Input: part model. Units: mm. Frame: model coordinates. Face numbers are marked on the shaded views. Coordinates: 2 decimals unless noted, no trailing zeros. Write each loop counter-clockwise with the first axis right and the second up, starting at its lowest first coordinate (ties: lowest second). Pieces come first, ordered by that corner, then holes. Notation, with made-up numbers: M 65.25,-0.75 L 100.25,-0.75 A11 cw 100.25,20.25 Z; hole C 8,-23 d9. An arc over 180 degrees is marked long. Use one line per item in the form item = value.
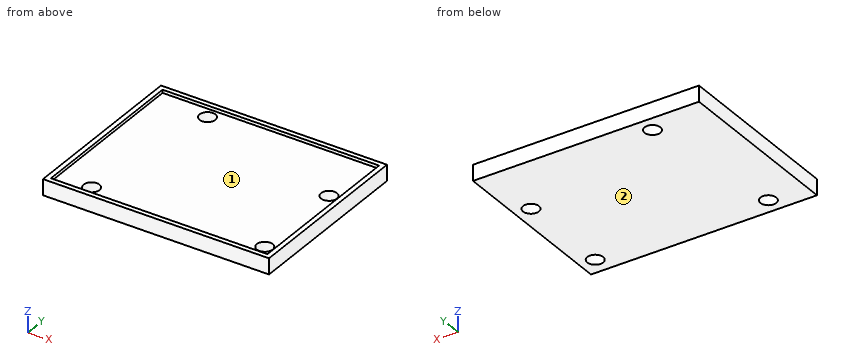
from build123d import *

# Parameters (mm, degrees)
SKETCH1_W           = 71.31
SKETCH1_H           = 56
BOSS_EXTRUDE1_DEPTH = 5
SKETCH2_R           = 2.5
CUT_EXTRUDE1_DEPTH  = 5
SKETCH3_W           = 68.31
SKETCH3_H           = 53
CUT_EXTRUDE2_DEPTH  = 1


with BuildPart() as part:
    # Sketch1 → Boss-Extrude1 (new body)
    with BuildSketch(Plane.XY):
        Rectangle(SKETCH1_W, SKETCH1_H)
    extrude(amount=BOSS_EXTRUDE1_DEPTH)

    # Sketch2 → Cut-Extrude1 (cut)
    with BuildSketch(Plane.XY.offset(5)):
        with Locations((-23.655, -23)):
            Circle(SKETCH2_R)
        with Locations((30.655, 8)):
            Circle(SKETCH2_R)
        with Locations((-17.655, 23)):
            Circle(SKETCH2_R)
        with Locations((30.655, -22.5)):
            Circle(SKETCH2_R)
    extrude(amount=-CUT_EXTRUDE1_DEPTH, mode=Mode.SUBTRACT)

    # Sketch3 → Cut-Extrude2 (cut)
    with BuildSketch(Plane.XY.offset(5)):
        Rectangle(SKETCH3_W, SKETCH3_H)
    extrude(amount=-CUT_EXTRUDE2_DEPTH, mode=Mode.SUBTRACT)


solid = part.part
(1) Section query D-D on y = 18. Return the cut outline in (x, z) (3 decimals), plus the area to 3 significant figures.
Computed:
outline = M -35.655,0 L 35.655,0 L 35.655,5 L 34.155,5 L 34.155,4 L -34.155,4 L -34.155,5 L -35.655,5 Z
area = 288 mm^2
(2) First-contact query: pin 1 Ø2 at (x, y) = (11, -15.5) entering from +Z. Flat tip, straight axial feed; report the tip coordinate or a pass-through.
Computed:
pin_1 = 4
(3) Section query B-B on x = -24. Return the cut outline in (y, z).
Computed:
outline = M -28,0 L -25.48,0 L -25.48,4 L -26.5,4 L -26.5,5 L -28,5 Z; M -20.52,0 L 28,0 L 28,5 L 26.5,5 L 26.5,4 L -20.52,4 Z
(4) Line query: probe 1 along Y at (x, z) = (-6, 4.4); probe 2 along X at (y, z) = (-21.5, 1.2) (3 decimals); probe 3 along Z at (x, y) = (29, -8). Output: solid intervals per line, ascending.
Computed:
probe_1 = -28 to -26.5, 26.5 to 28
probe_2 = -35.655 to -25.655, -21.655 to 28.364, 32.946 to 35.655
probe_3 = 0 to 4
(5) Section query C-C on z = 3.1. Return the cut outline in (x, y) (3 decimals), plus the area to 3 significant figures.
Computed:
outline = M -35.655,-28 L 35.655,-28 L 35.655,28 L -35.655,28 Z; hole C -23.655,-23 d5; hole C -17.655,23 d5; hole C 30.655,-22.5 d5; hole C 30.655,8 d5
area = 3,910 mm^2
(6) Pull-direction query (Y, two-part tool) for the marked faces 1 and 2; classes: pulls with the +Y half, pulls with the -Y half, needs draft (parallel to the pull), parting line crosses it, or undercut.
Computed:
face_1 = undercut
face_2 = needs draft
(7) Section query A-A on y = 8. Return the cut outline in (x, z) (3 decimals), plus the area to 3 significant figures.
Computed:
outline = M -35.655,0 L 28.155,0 L 28.155,4 L -34.155,4 L -34.155,5 L -35.655,5 Z; M 33.155,0 L 35.655,0 L 35.655,5 L 34.155,5 L 34.155,4 L 33.155,4 Z
area = 268 mm^2
